Print and shaded views of the part. All mm, measured from the part's lowest x, y and z. A direction names the side the tool comes from. Round coordinates to 2 decimals unless told otherwise and drop trailing zeros. Order: outer loops, then holes, each group sorted by start corner. A loop starts at its lowest first (then second) coordinate and runs counter-clockwise, first axis right, second up. Notation, with made-up numbers: M 66.5,-13.5 L 81.5,-13.5 A25 cw 81.5,8.5 Z; hole C 87,48 d9. An arc over 180 degrees is marked long. Use CSV: the item, a comma, the result in double quotes.
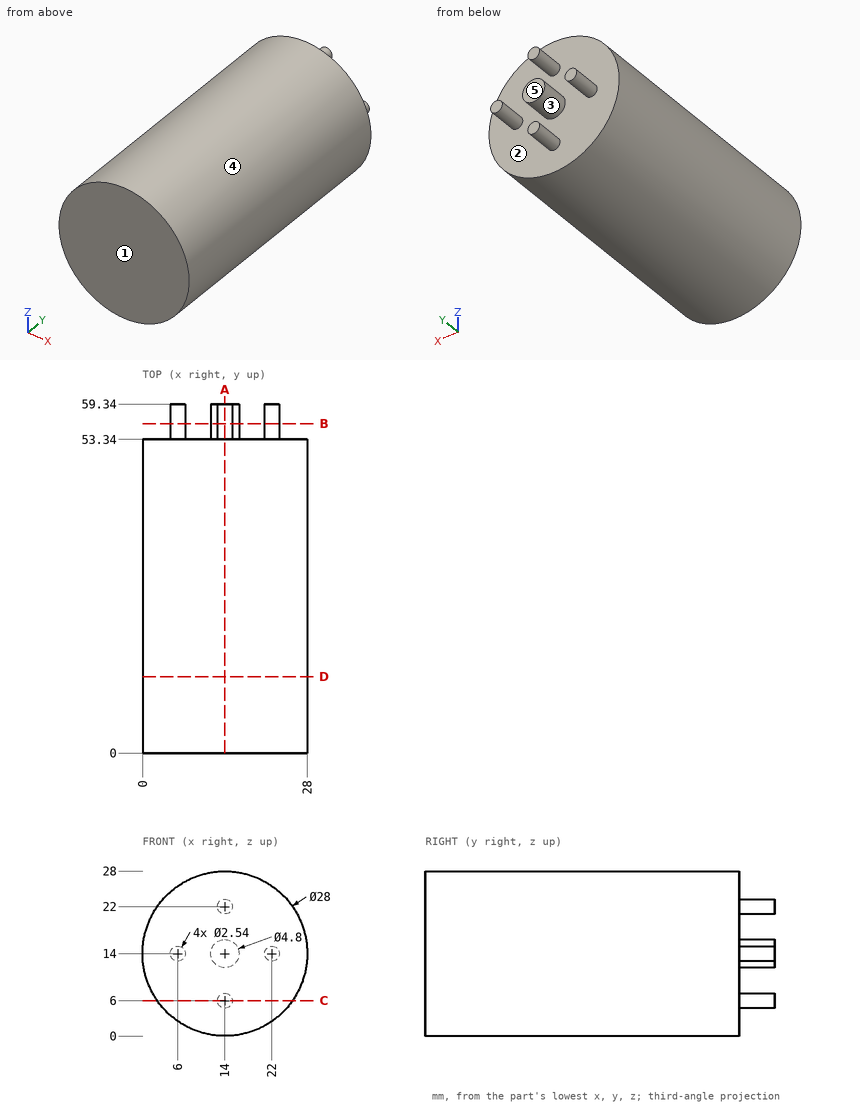
(1) Tool access for the marked faces 1 and 2: list every direction of +Z, -Z, +X, -X, +Y, -Y with a clear straight run to the whole face (end or side of a thin tool).
Answer block:
face 1,"+Z, -Z, +X, -X, -Y"
face 2,"+Y"
(2) Drop flat-ended pins along their axis: pin 1 (6 mm diameter, centred on x = 9, z = 16.5, fed in from -Y); pin 2 (8 mm diameter, centred on x = 7.5, y = 16.5, fed in from -Z) (3 decimals); pin 3 (1.5 mm diameter, centred on x = 12.5, z = 19.5, fed in from +Y); pin 4 (6 mm diameter, centred on x = 5.5, y = 32.5, fed in from +Z). Give the stop position or say it passes through.
Answer block:
pin 1,"stops at y = 0"
pin 2,"stops at z = 0.225"
pin 3,"stops at y = 53.34"
pin 4,"stops at z = 26.87"
(3) Two-plate mould, pull along Z, no slides. Class the marked faces 3, 4 and 5: released by +Z, released by -Z, zero draft, split by the parting line, or undercut.
Answer block:
face 3,"undercut"
face 4,"split by the parting line"
face 5,"zero draft"
(4) Cut at B-B, the plane y = 56. Give the cut face in (x, z), and give its area (3 significant figures).
Answer block:
outline,"C 6,14 d2.54; C 14,14 d4.8; C 14,6 d2.54; C 14,22 d2.54; C 22,14 d2.54"
area,"38.4 mm²"
(5) Wall check: line 1 (X direction, y = 43, z = 14.25); line 2 (Z direction, x = 14.5, y = 41); line 3 (Y direction, x = 3.25, z = 12.75). Give the ranges that are in metal, low to high. Write a range as from..to.
Answer block:
line 1,"x = 0..28"
line 2,"z = 0.01..27.99"
line 3,"y = 0..53.34"
(6) Cut at A-A, the plane x = 14. Give the cut face in (y, z), and give its area (3 significant figures).
Answer block:
outline,"M 0,0 L 53.34,0 L 53.34,4.73 L 59.34,4.73 L 59.34,7.27 L 53.34,7.27 L 53.34,11.6 L 59.34,11.6 L 59.34,16.4 L 53.34,16.4 L 53.34,20.73 L 59.34,20.73 L 59.34,23.27 L 53.34,23.27 L 53.34,28 L 0,28 Z"
area,"1,550 mm²"
(7) Cut at C-C, the plane z = 6. Give the cut face in (x, y).
Answer block:
outline,"M 2.51,0 L 25.49,0 L 25.49,53.34 L 15.27,53.34 L 15.27,59.34 L 12.73,59.34 L 12.73,53.34 L 2.51,53.34 Z"
(8) Cut at D-D, the plane y = 13. Give the cut face in (x, z), and give its area (3 significant figures).
Answer block:
outline,"C 14,14 d28"
area,"616 mm²"
